```python
from build123d import *

# Parameters (mm, degrees)
F0_R     = 21.336
F0_R_2   = 18.796
F1_DEPTH = 215.9
F5_START = -184.15
F5_DEPTH = 6.35


with BuildPart() as f1:
    # F0 (on Top) → F1 (new body)
    with BuildSketch(Plane.XY):
        Circle(F0_R)
        Circle(F0_R_2, mode=Mode.SUBTRACT)
    extrude(amount=-F1_DEPTH)

    # F2 (on Front) → F3 (revolve)
    with BuildSketch(Plane.XZ):
        Polygon((18.796, 0), (21.336, 0), (30.5808439504, 25.4), (28.0408439504, 25.4), align=None)
    revolve(axis=Axis((0, 0, 12.7485655248), (0, 0, 1)))

    # F4 (on Top) → F5 (join)
    with BuildSketch(Plane.XY.offset(F5_START)):
        with BuildLine():
            Line((-23.7851446116, -2.0809305138), (-21.2548100785, -1.8595549273))
            ThreePointArc((-21.2548100785, -1.8595549273), (-21.336, 0), (-21.2548100785, 1.8595549273))
            Line((-21.2548100785, 1.8595549273), (-23.7851446116, 2.0809305138))
            ThreePointArc((-23.7851446116, 2.0809305138), (-23.876, 0), (-23.7851446116, -2.0809305138))
        make_face()
        with BuildLine():
            Line((-2.0809305138, 23.7851446116), (-1.8595549273, 21.2548100785))
            ThreePointArc((-1.8595549273, 21.2548100785), (0, 21.336), (1.8595549273, 21.2548100785))
            Line((1.8595549273, 21.2548100785), (2.0809305138, 23.7851446116))
            ThreePointArc((2.0809305138, 23.7851446116), (0, 23.876), (-2.0809305138, 23.7851446116))
        make_face()
        with BuildLine():
            Line((23.7851446116, 2.0809305138), (21.2548100785, 1.8595549273))
            ThreePointArc((21.2548100785, 1.8595549273), (21.336, 0), (21.2548100785, -1.8595549273))
            Line((21.2548100785, -1.8595549273), (23.7851446116, -2.0809305138))
            ThreePointArc((23.7851446116, -2.0809305138), (23.876, 0), (23.7851446116, 2.0809305138))
        make_face()
        with BuildLine():
            Line((2.0809305138, -23.7851446116), (1.8595549273, -21.2548100785))
            ThreePointArc((1.8595549273, -21.2548100785), (0, -21.336), (-1.8595549273, -21.2548100785))
            Line((-1.8595549273, -21.2548100785), (-2.0809305138, -23.7851446116))
            ThreePointArc((-2.0809305138, -23.7851446116), (0, -23.876), (2.0809305138, -23.7851446116))
        make_face()
    extrude(amount=-F5_DEPTH)

    # F6 (on Front) → F7 (revolve, cut)
    with BuildSketch(Plane.XZ):
        Polygon((23.876, -186.1005909488), (21.336, -190.5), (23.876, -190.5), align=None)
    revolve(axis=Axis((0, 0, -83.1778421998), (0, 0, -1)), mode=Mode.SUBTRACT)


solid = f1.part
```
Source: CAD feature listing. Evaluate the final solid. Frame: model axes, mm. Coordinates: 2 decimals unless noted, no trailing zeros. Loops run counter-clockwise (first coordinate to the right, second up) from the corner with the lowest first, then second, coordinate; pieces in that order, holes last. Notation, with made-up numbers: M 25.25,3 L 37.25,3 A28 cw 37.25,35 Z; hole C 69.25,14 d6. An arc over 180 degrees is marked long. Use a Markdown table: item, result. Add a question column.
Q1. Draft query along X for faces 1 (the conical face through (-22.59, -0.03, -188.33)), 2 (the cylindrical face through (-2.447, 18.636, -106.439)), 3 (the flat face through (13.45, -24.78, 25.4)). Return one class per face: pulls with the +X half, pulls with the -X half, needs draft (parallel to the pull), parting line crosses it, or undercut.
Q2. Material intervals for L1, parallel to Y at x = -1, z = -197; L2, parallel to X at y = -12.5, z = -27; L3, parallel to X at y = 4, z = -69.5, sorted ascending.
Q3. Section query A-A, the plane z = -65. Return loops of the section in (x, y).
Q4. First-contact query: pin 1 (12 mm diameter, centred on y = -11, z = -178, fed in from -X); pin 2 (6 mm diameter, centred on y = 12, z = -80.5, fed in from +X); pin 3 (2 mm diameter, centred on y = -1, z = -36, fed in from +X). Flat tips, straight axial feed; report the tip coordinate or a pass-through.
Result:
| question | item | result |
|---|---|---|
| 1 | face 1 | pulls with the -X half |
| 1 | face 2 | undercut |
| 1 | face 3 | needs draft |
| 2 | L1 | y = -21.31 to -18.77, 18.77 to 21.31 |
| 2 | L2 | x = -17.29 to -14.04, 14.04 to 17.29 |
| 2 | L3 | x = -20.96 to -18.37, 18.37 to 20.96 |
| 3 | outline | C 0,0 d42.67; hole C 0,0 d37.59 |
| 4 | pin 1 | stops at x = -20.74 |
| 4 | pin 2 | stops at x = 19.34 |
| 4 | pin 3 | stops at x = 21.34 |
